The figure shows three views and two pictorial views of one solid part (mm, origin at its lowest corner). Answer the questions. A direction names the side the tool comes from. Give positions to 0.01 mm unless a question says otherwise; leave off trailing zeros. Write each loop counter-clockwise with the first axis right and the second up, starting at its lowest first coordinate (ties: lowest second). Pieces come first, ordered by that corner, then holes. Notation, with made-up numbers: (12, -16) - (17, -16) arc R12 ccw to (17, -6) - close; hole circle Ø3 at (72, -32). An arc over 180 degrees is marked (long way). Answer as CSV lines item,"result". Start each with the question number.
(1) For a pull along Z with two mould halves and no side action, classify the marked faces 1, 2 and 3 as pulls with the +Z half, pulls with the -Z half, needs draft (parallel to the pull), parting line crosses it, or undercut.
(2) Find section C-C (y = 8). Write down the section's boundary in (x, z).
(3) Straight lines are drawn through the part: probe 1 along X at (y, z) = (8.55, 2.9); probe 2 along Y at (x, z) = (2.55, 1.5). For each, find the intervals that lie inside material, in ascending order.
(4) For the marked faces 4 and 5, determine the directions among +Z, -Z, +X, -X, +Y, -Y from which every point of the face is accessible in a straight line to the end or side of a thin tool.
(5) Find section B-B (x = 2.9). Write down the section's boundary in (y, z).
(6) Each of these flat-tipped pins is pushed along its axis until it touches: pin 1 Ø1.5 at (x, z) = (3, 2.5) entering from +Y; pin 2 Ø2 at (y, z) = (6.5, 1) entering from +X; pin 3 Ø2 at (x, z) = (1, 5) entering from -Y. Where does it stop, or does it pass through?
(7) Find section A-A (z = 2.9). Write down the section's boundary in (x, y), then the cut area to 3 significant figures.
(8) Find section D-D (y = 1.5). Write down the section's boundary in (x, z), then the cut area to 3 significant figures.
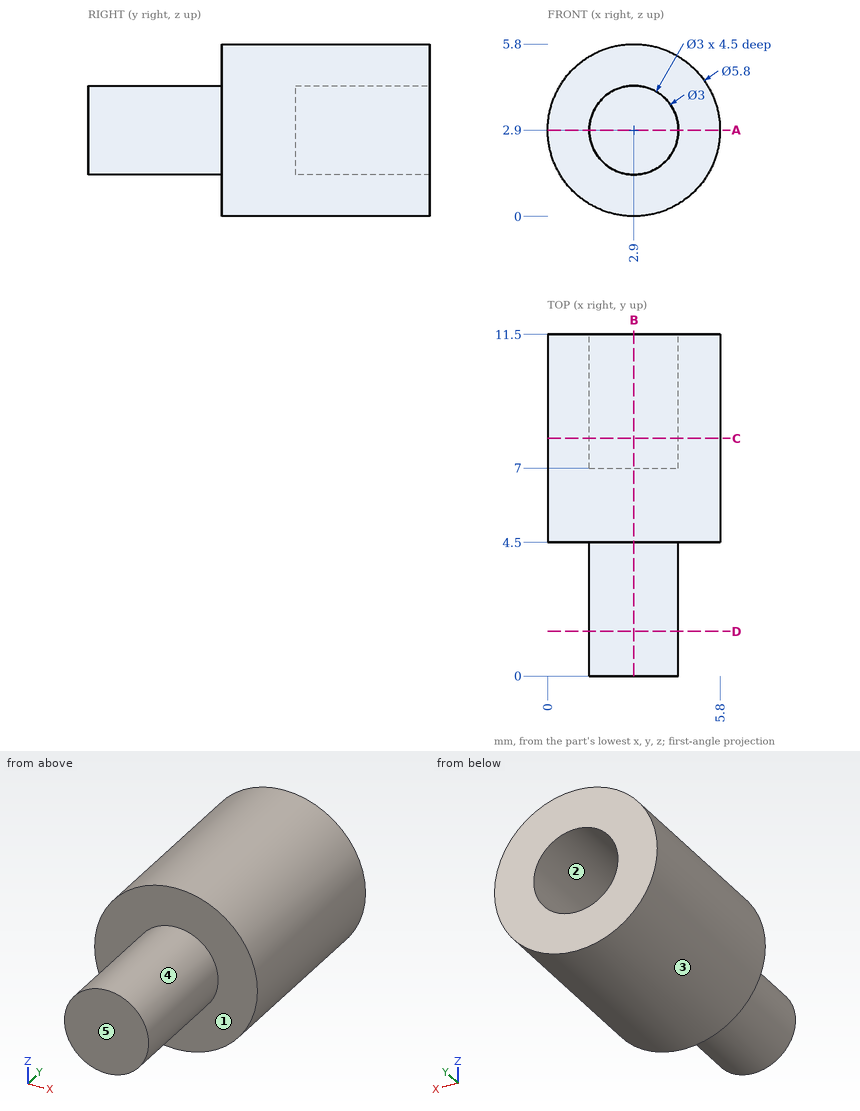
Result set:
1,face 1,"needs draft"
1,face 2,"undercut"
1,face 3,"parting line crosses it"
2,outline,"circle Ø5.8 at (2.9, 2.9); hole circle Ø3 at (2.9, 2.9)"
3,probe 1,"0 to 1.4, 4.4 to 5.8"
3,probe 2,"0 to 7"
4,face 4,"-Y"
4,face 5,"+Z, -Z, +X, -X, -Y"
5,outline,"(0, 1.4) - (4.5, 1.4) - (4.5, 0) - (11.5, 0) - (11.5, 1.4) - (7, 1.4) - (7, 4.4) - (11.5, 4.4) - (11.5, 5.8) - (4.5, 5.8) - (4.5, 4.4) - (0, 4.4) - close"
6,pin 1,"y = 7"
6,pin 2,"x = 5.66"
6,pin 3,"y = 4.5"
7,outline,"(0, 4.5) - (1.4, 4.5) - (1.4, 0) - (4.4, 0) - (4.4, 4.5) - (5.8, 4.5) - (5.8, 11.5) - (4.4, 11.5) - (4.4, 7) - (1.4, 7) - (1.4, 11.5) - (0, 11.5) - close"
7,area,"40.6 mm^2"
8,outline,"circle Ø3 at (2.9, 2.9)"
8,area,"7.07 mm^2"
